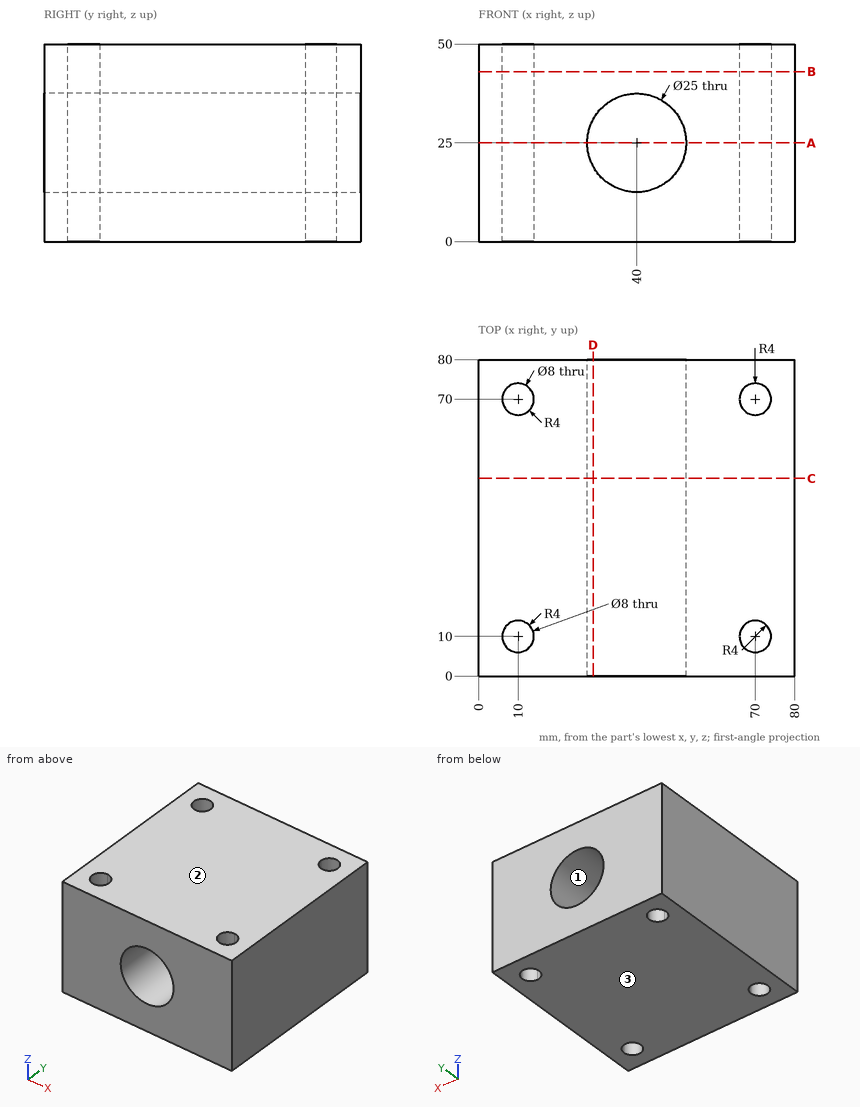
For this review, use the dimensioned drawing (mm, ordinates from the lowest corner) and the shaded views. Round coordinates to 2 decimals unless told otherwise and drop trailing zeros. Write each loop counter-clockwise with the first axis right and the second up, starting at its lowest first coordinate (ties: lowest second). Pieces come first, ordered by that corner, then holes. Notation, with made-up numbers: (69.25, 67.5) -> (76.25, 67.5) arc R20 cw to (76.25, 89.5) -> close; hole circle Ø9 at (-36.75, 43). An arc over 180 degrees is marked (long way). Answer in a Markdown table with one row per item.
Q1. Take a section at C-C, the plane y = 50. State the section outline as (x, z) points.
The answers:
| item | result |
|---|---|
| outline | (0, 0) -> (80, 0) -> (80, 50) -> (0, 50) -> close; hole circle Ø25 at (40, 25) |
Q2. Take a section at B-B, the plane z = 43. State the section outline as (x, y) points, then the cut area to 3 significant figures.
The answers:
| item | result |
|---|---|
| outline | (0, 0) -> (80, 0) -> (80, 80) -> (0, 80) -> close; hole circle Ø8 at (10, 10); hole circle Ø8 at (10, 70); hole circle Ø8 at (70, 10); hole circle Ø8 at (70, 70) |
| area | 6,200 mm² |
Q3. Clearance check with a flat-ended pin moving along its axis: pin 1 Ø6 at (x, y) = (47.5, 17.5) entering from -Z. State where the tip first meets the part, or that it passes through.
The answers:
| item | result |
|---|---|
| pin 1 | z = 0 |
Q4. Take a section at D-D, the plane x = 29. State the section outline as (y, z) points.
The answers:
| item | result |
|---|---|
| outline | (0, 0) -> (80, 0) -> (80, 19.06) -> (0, 19.06) -> close; (0, 30.94) -> (80, 30.94) -> (80, 50) -> (0, 50) -> close |
Q5. Draft analysis for pull direction Z (two halves, no side actions). For the marked faces 1, 2 and 3, state which applies: +Z half, -Z half, draft (parallel to the pull), parting line (faces both ways), or undercut.
The answers:
| item | result |
|---|---|
| face 1 | undercut |
| face 2 | +Z half |
| face 3 | -Z half |
Q6. To check wall thickness, follow L1, parallel to Y at x = 10, z = 15.5; L2, parallel to X at y = 70, z = 13.5; L3, parallel to X at y = 13, z = 30.5. State the ranges of each line that lie inside material, in increasing order. Write a range as [from, to].
The answers:
| item | result |
|---|---|
| L1 | [0, 6], [14, 66], [74, 80] |
| L2 | [0, 6], [14, 35.1], [44.9, 66], [74, 80] |
| L3 | [0, 7.35], [12.65, 28.78], [51.22, 67.35], [72.65, 80] |
Q7. Take a section at A-A, the plane z = 25. State the section outline as (x, y) points.
The answers:
| item | result |
|---|---|
| outline | (0, 0) -> (27.5, 0) -> (27.5, 80) -> (0, 80) -> close; (52.5, 0) -> (80, 0) -> (80, 80) -> (52.5, 80) -> close; hole circle Ø8 at (10, 10); hole circle Ø8 at (10, 70); hole circle Ø8 at (70, 10); hole circle Ø8 at (70, 70) |
